Can you work these out from the drawing? Everything is in mm from the part's minimum corner. A direction names the side the tool comes from. Coordinates: 2 decimals unless noted, no trailing zeros. Write each loop counter-clockwise with the first axis right and the second up, starting at its lowest first coordinate (ties: lowest second). Pieces come first, ordered by that corner, then holes. Notation, with made-up numbers: (76.25, -21.75) -> (87.25, -21.75) arc R18 cw to (87.25, 1.25) -> close; hole circle Ø2 at (-7.75, 65.25). An arc over 180 degrees is marked (long way). Use a Markdown table: item, result. Add a question column.
Item 1: If I drill on line 1 along X through (y, z) = (11, 4.25); line 2 along Z through (x, y) = (41.5, 5.75); line 3 along Z through (x, y) = (43, 3.5), over which ranges is the centre line in solid material (lowest first)? Write a range as from..to.
Item 2: Imagine slicing it at C-C, the plane x = 34.5. Write out the boundary of the cut face in (y, z).
Item 3: Imagine slicing it at A-A, the plane y = 6. Write out the boundary of the cut face in (x, z).
Item 4: On a 3-axis mill with a long thin cutter (end or side, diameter ignored), from which of +Z, -Z, +X, -X, +Y, -Y can I reach the whole of each face in a straight line? I mean the marked faces 1, 2 and 3. Say none if no direction works.
Item 5: Will these pins go through, and if not, where does the flat tip stop? pin 1 Ø2 at (x, y) = (40.5, 9.5) entering from +Z; pin 2 Ø2 at (x, z) = (49.5, 1.5) entering from +Y; pin 3 Ø4 at (y, z) = (1.5, 8) entering from -X; pin 4 Ø3 at (x, y) = (45, 3) entering from -Z.
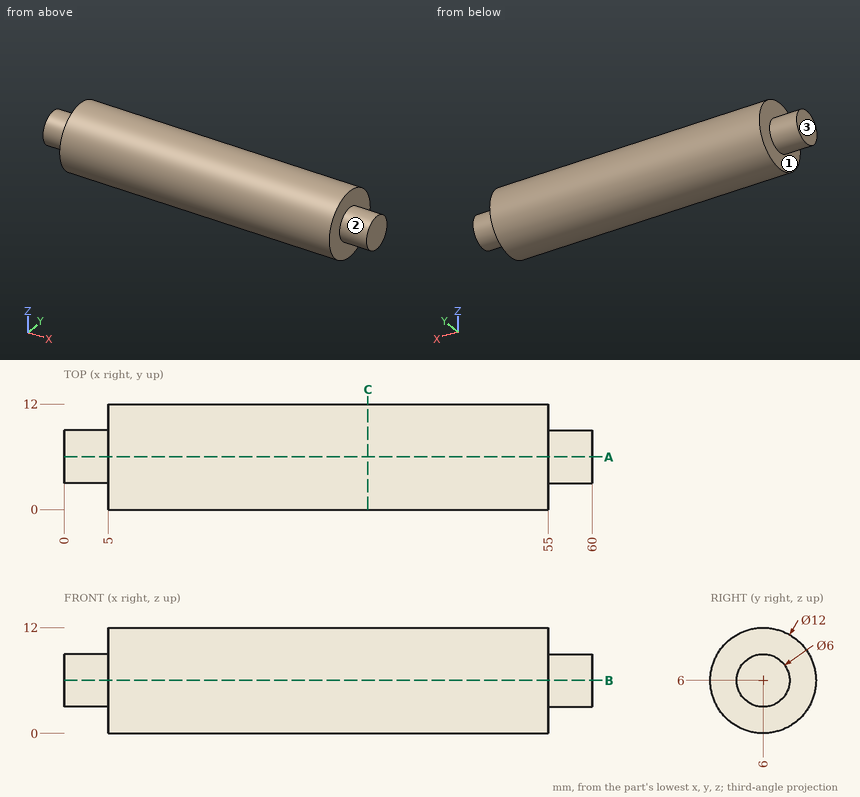
Ans:
| question | item | result |
|---|---|---|
| 1 | line 1 | x = 5..55 |
| 1 | line 2 | z = 0.01..11.99 |
| 1 | line 3 | z = 0.55..11.45 |
| 2 | outline | circle Ø12 at (6, 6) |
| 3 | outline | (0, 3) -> (5, 3) -> (5, 0) -> (55, 0) -> (55, 3) -> (60, 3) -> (60, 9) -> (55, 9) -> (55, 12) -> (5, 12) -> (5, 9) -> (0, 9) -> close |
| 4 | face 1 | -X |
| 4 | face 2 | +X |
| 4 | face 3 | +Z, -Z, -X, +Y, -Y |
| 5 | pin 1 | stops at z = 11.45 |
| 5 | pin 2 | stops at y = 10.87 |
| 5 | pin 3 | stops at x = 0 |
| 5 | pin 4 | stops at z = 0.19 |
